Here's how the part is built. I have some questions about the finished solid (model axes, mm). A direction names the side the tool comes from. Coordinates: 2 decimals unless noted, no trailing zeros. Write each loop counter-clockwise with the first axis right and the second up, starting at its lowest first coordinate (ties: lowest second). Pieces come first, ordered by that corner, then holes. Notation, with made-up numbers: M -28.5,-28 L -16.5,-28 A27 cw -16.5,-3 Z; hole C -7.75,44.5 d5. An arc over 180 degrees is marked long. Use a Markdown table: item, result.
```python
from build123d import *

# Parameters (mm, degrees)
BASE_FLANGE1_DEPTH            = 1
EDGE_FLANGE1_STRIP_W          = 5
EDGE_FLANGE1_STRIP_H          = 1
EDGE_FLANGE1_STRIP_CUT_DEPTH  = 169
EDGE_FLANGE1_RELIEF_W         = 5.5
EDGE_FLANGE1_RELIEF_H         = 0.5
EDGE_FLANGE1_RELIEF_CUT_DEPTH = 1
EDGE_FLANGE1_DEPTH            = 169
EDGE_FLANGE2_STRIP_W          = 5
EDGE_FLANGE2_STRIP_H          = 1
EDGE_FLANGE2_STRIP_CUT_DEPTH  = 169
EDGE_FLANGE2_DEPTH            = 169
SKETCH12_R                    = 1.5
CUT_EXTRUDE1_DEPTH            = 3


# Sheet-metal steps are written as plain solids
with BuildPart() as part:
    # Sketch1 → Base-Flange1 (new body)
    with BuildSketch(Plane(origin=(0, 0, 0), x_dir=(1, 0, 0), z_dir=(0, 1, 0))):
        Polygon((-84.5, 0), (84.5, 0), (94.5, 10), (-84.5, 10), align=None)
    extrude(amount=-BASE_FLANGE1_DEPTH)

    # Edge-Flange1 strip (across the edge) → Edge-Flange1 strip cut (cut)
    with BuildSketch(Plane(origin=(84.5, -1, 0), x_dir=(0, 0, -1), z_dir=(-1, 0, 0))):
        with Locations((-2, -0.5)):
            Rectangle(EDGE_FLANGE1_STRIP_W, EDGE_FLANGE1_STRIP_H)
    extrude(amount=EDGE_FLANGE1_STRIP_CUT_DEPTH, mode=Mode.SUBTRACT)

    # Edge-Flange1 relief (on the sheet) → Edge-Flange1 relief cut (cut)
    with BuildSketch(Plane(origin=(84.5, -1, -0.5), x_dir=(0, 0, -1), z_dir=(0, -1, 0))):
        with Locations((-2.25, 0.25)):
            Rectangle(EDGE_FLANGE1_RELIEF_W, EDGE_FLANGE1_RELIEF_H)
    extrude(amount=-EDGE_FLANGE1_RELIEF_CUT_DEPTH, mode=Mode.SUBTRACT)

    # Edge-Flange1 section (across the edge) → Edge-Flange1 (add)
    with BuildSketch(Plane(origin=(84.5, -1, 0), x_dir=(0, 0, -1), z_dir=(-1, 0, 0))):
        with BuildLine():
            Line((-1, 0.5), (-1, 7))
            Line((-1, 7), (0, 7))
            Line((0, 7), (0, 0.5))
            ThreePointArc((0, 0.5), (0.146446609, 0.146446609), (0.5, 0))
            Line((0.5, 0), (0.5, -1))
            ThreePointArc((0.5, -1), (-0.560660172, -0.560660172), (-1, 0.5))
        make_face()
    extrude(amount=EDGE_FLANGE1_DEPTH)

    # Edge-Flange2 strip (across the edge) → Edge-Flange2 strip cut (cut)
    with BuildSketch(Plane(origin=(84.5, -8, 0), x_dir=(0, 1, 0), z_dir=(-1, 0, 0))):
        with Locations((-2, -0.5)):
            Rectangle(EDGE_FLANGE2_STRIP_W, EDGE_FLANGE2_STRIP_H)
    extrude(amount=EDGE_FLANGE2_STRIP_CUT_DEPTH, mode=Mode.SUBTRACT)

    # Edge-Flange2 section (across the edge) → Edge-Flange2 (add)
    with BuildSketch(Plane(origin=(84.5, -8, 0), x_dir=(0, 1, 0), z_dir=(-1, 0, 0))):
        with BuildLine():
            Line((-1, 0.5), (-1, 9))
            Line((-1, 9), (0, 9))
            Line((0, 9), (0, 0.5))
            ThreePointArc((0, 0.5), (0.146446609, 0.146446609), (0.5, 0))
            Line((0.5, 0), (0.5, -1))
            ThreePointArc((0.5, -1), (-0.560660172, -0.560660172), (-1, 0.5))
        make_face()
    extrude(amount=EDGE_FLANGE2_DEPTH)

    # Sketch12 → Cut-Extrude1 (cut)
    with BuildSketch(Plane.XZ.offset(9)):
        with Locations(Location((-74.5, -5, 0), (0, 0, 270))):
            Circle(SKETCH12_R)
        with Locations(Location((0, -5, 0), (0, 0, 270))):
            Circle(SKETCH12_R)
        with Locations(Location((74.5, -5, 0), (0, 0, 270))):
            Circle(SKETCH12_R)
    extrude(amount=-CUT_EXTRUDE1_DEPTH, mode=Mode.SUBTRACT)


solid = part.part
```
1. Suppose I cut it at B-B on x = 0. Write out the boundary of the cut face in (y, z), and give its area (3 significant figures).
Answers follow:
| item | result |
|---|---|
| outline | M -9,-9 L -8,-9 L -8,-6.5 L -9,-6.5 Z; M -9,-3.5 L -8,-3.5 L -8,-0.5 A0.5 cw -7.5,0 L -1.5,0 A0.5 cw -1,-0.5 L -1,-10 L 0,-10 L 0,-0.5 A1.5 ccw -1.5,1 L -7.5,1 A1.5 ccw -9,-0.5 Z |
| area | 24.1 mm2 |
2. We'd pull the mould along X, two halves only. Please class faces 4 (the face through (-84.5, -0.8, -3.3)), 5 (the face through (1, -8, -3)), 6 (the face through (89.7, -0.5, -5.2)), 7 (the face through (-73.235, -8.507, -5.806)): +X half, -X half, draft (parallel to the pull), parting line (faces both ways), or undercut.
Answers follow:
| item | result |
|---|---|
| face 4 | -X half |
| face 5 | draft |
| face 6 | +X half |
| face 7 | undercut |
3. Which directions (+Z, -Z, +X, -X, +Y, -Y) give clear straight access to the entire face, cutting with the end or side of a thin tool? Please do faces 1 (the face through (4, -1, -5)), 2 (the face through (1.2, -9, -3.7)), 3 (the face through (75.765, -8.507, -5.806)).
Answers follow:
| item | result |
|---|---|
| face 1 | -Z, +X, -X |
| face 2 | +Z, -Z, +X, -X, -Y |
| face 3 | -Y |
4. Suppose I cut it at A-A on z = -5. Write out the boundary of the cut face in (x, y).
Answers follow:
| item | result |
|---|---|
| outline | M -84.5,-9 L -76,-9 L -76,-8 L -84.5,-8 Z; M -84.5,-1 L 89.5,-1 L 89.5,0 L -84.5,0 Z; M -73,-9 L -1.5,-9 L -1.5,-8 L -73,-8 Z; M 1.5,-9 L 73,-9 L 73,-8 L 1.5,-8 Z; M 76,-9 L 84.5,-9 L 84.5,-8 L 76,-8 Z |
5. Will these pins go through, and if not, where does the flat tip stop? pin 1 Ø2.5 at (x, z) = (41, -6) entering from +Y; pin 2 Ø1 at (y, z) = (-2, -1) entering from +X; pin 3 Ø2.5 at (x, z) = (74.5, -5) entering from -Y.
Answers follow:
| item | result |
|---|---|
| pin 1 | stops at y = 0 |
| pin 2 | passes through |
| pin 3 | stops at y = -1 |
6. I need wall thicknesses on probe 1 along X at (y, z) = (-8.55, -5); probe 2 along Y at (x, z) = (32, -2.5); probe 3 along Z at (x, y) = (74.5, -8.55). Which ranges of each line are inside material? Lowest first, please.
Answers follow:
| item | result |
|---|---|
| probe 1 | x = -84.5 to -76, -73 to -1.5, 1.5 to 73, 76 to 84.5 |
| probe 2 | y = -9 to -8, -1 to 0 |
| probe 3 | z = -9 to -6.5, -3.5 to 0.57 |
